from build123d import *

# Parameters (mm, degrees)
SKETCH1_W                              = 196
SKETCH1_H                              = 96
EXTRUDE1_DEPTH                         = 12
CBORE_FOR_10_MM_CORE_PINS1_D           = 10.5
CBORE_FOR_10_MM_CORE_PINS1_CBORE_D     = 16
CBORE_FOR_10_MM_CORE_PINS1_CBORE_DEPTH = 5
CBORE_FOR_5_MM_CORE_PINS1_D            = 5.3
CBORE_FOR_5_MM_CORE_PINS1_CBORE_D      = 11
CBORE_FOR_5_MM_CORE_PINS1_CBORE_DEPTH  = 3
CBORE_FOR_8_MM_CORE_PINS1_D            = 8.3
CBORE_FOR_8_MM_CORE_PINS1_CBORE_D      = 15
CBORE_FOR_8_MM_CORE_PINS1_CBORE_DEPTH  = 5
F_20_0_20_DIAMETER_HOLE1_D             = 18
F_20_0_20_DIAMETER_HOLE1_DEPTH         = 12
F_20_0_20_DIAMETER_HOLE1_TIP           = 5.407745571


with BuildPart() as part:
    # Sketch1 → Extrude1 (new body)
    with BuildSketch(Plane.XY):
        Rectangle(SKETCH1_W, SKETCH1_H)
    extrude(amount=-EXTRUDE1_DEPTH)

    # CBORE for 10 mm Core Pins1 (through all)
    with Locations(Plane(origin=(0, 0, -12), x_dir=(-1, 0, 0), z_dir=(0, 0, -1))):
        with Locations((-85, 36), (85, 36), (85, -36), (-85, -36)):
            CounterBoreHole(CBORE_FOR_10_MM_CORE_PINS1_D / 2, CBORE_FOR_10_MM_CORE_PINS1_CBORE_D / 2, CBORE_FOR_10_MM_CORE_PINS1_CBORE_DEPTH)

    # CBORE for 5 mm Core Pins1 (through all)
    with Locations(Plane(origin=(0, 0, -12), x_dir=(-1, 0, 0), z_dir=(0, 0, -1))):
        with Locations((47, 10.939957651), (80, 10.939957651), (80, -10.939957651), (47, -10.939957651), (-47, 10.939957651), (-47, -10.939957651), (-80, 10.939957651), (-80, -10.939957651)):
            CounterBoreHole(CBORE_FOR_5_MM_CORE_PINS1_D / 2, CBORE_FOR_5_MM_CORE_PINS1_CBORE_D / 2, CBORE_FOR_5_MM_CORE_PINS1_CBORE_DEPTH)

    # CBORE for 8 mm Core Pins1 (through all)
    with Locations(Plane(origin=(0, 0, -12), x_dir=(-1, 0, 0), z_dir=(0, 0, -1))):
        with Locations((0, 0)):
            CounterBoreHole(CBORE_FOR_8_MM_CORE_PINS1_D / 2, CBORE_FOR_8_MM_CORE_PINS1_CBORE_D / 2, CBORE_FOR_8_MM_CORE_PINS1_CBORE_DEPTH)

    # Ø20.0 (20) Diameter Hole1
    with Locations(Plane(origin=(0, 0, -12), x_dir=(-1, 0, 0), z_dir=(0, 0, -1))):
        with Locations((-60, 30), (60, 30), (60, -30), (-60, -30)):
            Hole(F_20_0_20_DIAMETER_HOLE1_D / 2, depth=F_20_0_20_DIAMETER_HOLE1_DEPTH)
            with Locations((0, 0, -(F_20_0_20_DIAMETER_HOLE1_DEPTH + F_20_0_20_DIAMETER_HOLE1_TIP / 2))):  # 118° drill point
                Cone(0, F_20_0_20_DIAMETER_HOLE1_D / 2, F_20_0_20_DIAMETER_HOLE1_TIP, mode=Mode.SUBTRACT)


solid = part.part
Design review of the part built by this model. Coordinates are the model's own, in mm. A direction names the side the tool comes from. Give positions to 0.01 mm unless a question says otherwise; leave off trailing zeros. Order: outer loops, then holes, each group sorted by start corner. A loop starts at its lowest first (then second) coordinate and runs counter-clockwise, first axis right, second up. Notation, with made-up numbers: (82, 56) - (120, 56) arc R11 ccw to (120, 67) - close; hole circle Ø5 at (87.25, -19.5). An arc over 180 degrees is marked (long way). Write item = value, one per line. Start each with the question number.
Q1. Mouldability with a two-part tool opening along Y and no side actions: class faces 1 (the face through (-44, -12, -9)), 2 (the face through (98, -1, -6)) as released by +Y, released by -Y, zero draft, split by the parting line, or undercut.
Q2. To check wall thickness, follow L1, parallel to Y at x = -47, z = -3.25; L2, parallel to X at y = -30, z = -5.5; L3, parallel to Y at x = 80, z = -11.15 (3 decimals). State the ranges of each line that lie inside material, in increasing order. Write a range as from..to.
Q3. We need section C-C on y = -33. State the section outline as (x, z) points.
Q4. Clearance check with flat-ended pins moving along their axes: pin 1 Ø20.5 at (x, y) = (-60, 30) entering from -Z; pin 2 Ø4 at (x, y) = (80, -10.94) entering from -Z; pin 3 Ø5.5 at (x, y) = (79, -12.5) entering from -Z; pin 4 Ø5 at (x, y) = (88, 40) entering from -Z. State where each tip first meets the part, or that it passes through.
Q5. Tool access review of faces 3 (the face through (-47.574, -13.527, -4.437)), 4 (the face through (-90.2, 34.3, -7)): name each direction out of +Z, -Z, +X, -X, +Y, -Y from which nothing blocks a thin tool from reaching the whole face with its end or side.
Q6. We need section B-B on x = 47. State the section outline as (y, z) points, plus the area to 3 significant figures.
Q7. We need section A-A on y = 0. State the section outline as (x, z) points.
Q8. We need section D-D on z = -3.75. State how many separate pieces and enclosed holes the cut face has, plus the area to 3 significant figures.
Working result:
q1.face_1 = undercut
q1.face_2 = zero draft
q2.L1 = -48..-13.59, -8.29..8.29, 13.59..48
q2.L2 = -98..-69, -51..51, 69..98
q2.L3 = -48..-42.245, -29.755..-16.44, -5.44..5.44, 16.44..29.755, 42.245..48
q3.outline = (-98, -12) - (-92.42, -12) - (-92.42, -7) - (-89.31, -7) - (-89.31, 0) - (-98, 0) - close; (-80.69, -7) - (-77.58, -7) - (-77.58, -12) - (-68.49, -12) - (-68.49, 0) - (-80.69, 0) - close; (-51.51, -12) - (51.51, -12) - (51.51, 0) - (-51.51, 0) - close; (68.49, -12) - (77.58, -12) - (77.58, -7) - (80.69, -7) - (80.69, 0) - (68.49, 0) - close; (89.31, -7) - (92.42, -7) - (92.42, -12) - (98, -12) - (98, 0) - (89.31, 0) - close
q4.pin_1 = -12
q4.pin_2 = through
q4.pin_3 = -9
q4.pin_4 = -7
q5.face_3 = +Z, -Z
q5.face_4 = -Z
q6.outline = (-48, -12) - (-16.44, -12) - (-16.44, -9) - (-13.59, -9) - (-13.59, 0) - (-48, 0) - close; (-8.29, -9) - (-5.44, -9) - (-5.44, -12) - (5.44, -12) - (5.44, -9) - (8.29, -9) - (8.29, 0) - (-8.29, 0) - close; (13.59, -9) - (16.44, -9) - (16.44, -12) - (48, -12) - (48, 0) - (13.59, 0) - close
q6.area = 991 mm²
q7.outline = (-98, -12) - (-7.5, -12) - (-7.5, -7) - (-4.15, -7) - (-4.15, 0) - (-98, 0) - close; (4.15, -7) - (7.5, -7) - (7.5, -12) - (98, -12) - (98, 0) - (4.15, 0) - close
q8.separate_pieces = 1
q8.enclosed_holes = 17
q8.area = 17,200 mm²
